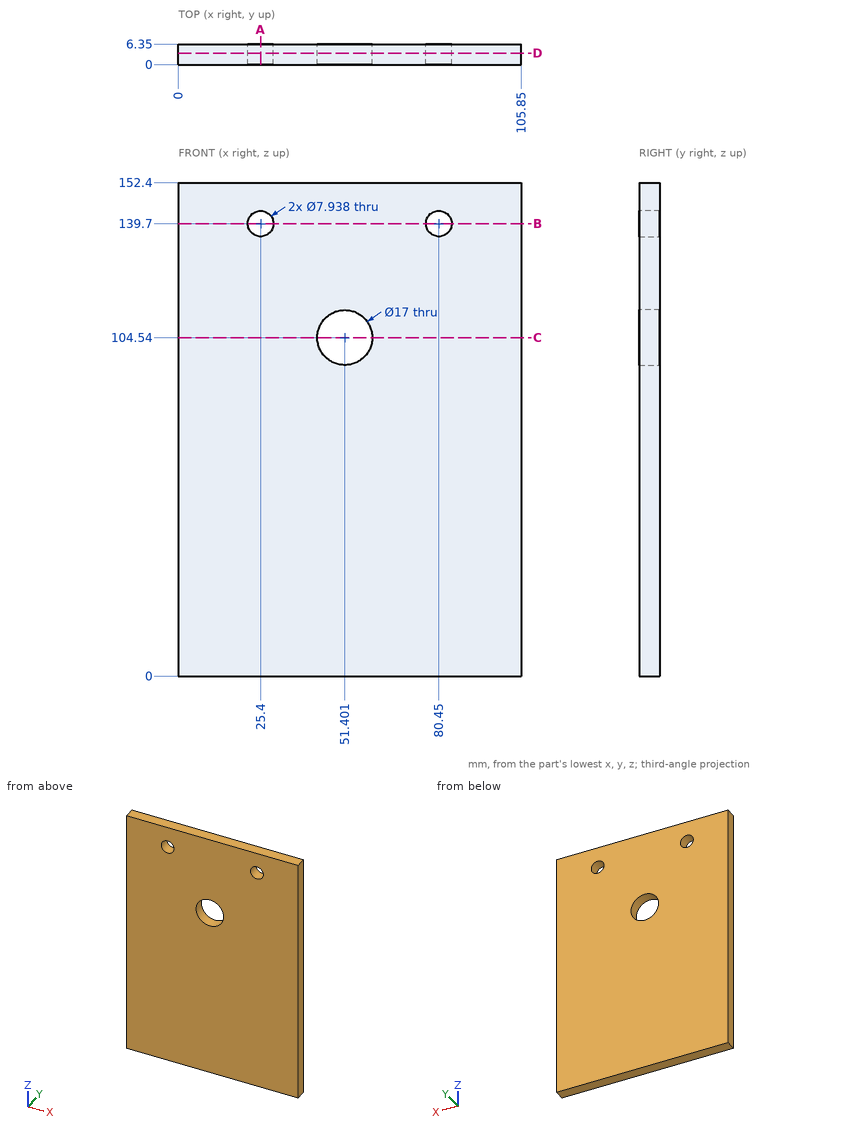
For this review, use the dimensioned drawing (mm, ordinates from the lowest corner) and the shaded views. Give positions to 0.01 mm unless a question says otherwise; leave off trailing zeros. Order: outer loops, then holes, each group sorted by start corner. A loop starts at its lowest first (then second) coordinate and runs counter-clockwise, first axis right, second up.
1) Take a section at B-B (z = 139.7). Give the boundary of the cut face in (x, y).
2) Take a section at C-C (z = 104.54). Give the boundary of the cut face in (x, y), then the cut area to 3 significant figures.
3) Take a section at D-D (y = 3.5). Give the boundary of the cut face in (x, z).
4) Take a section at A-A (x = 25.4). Give the boundary of the cut face in (y, z).
5) Wall thickness on line 1 (X direction, y = 4.25, z = 139.7); line 2 (X direction, y = 2.25, z = 104.54); line 3 (Z direction, x = 80.45, y = 4.5): over which ranges is each line inside the solid? List them lowest first.
6) Insertion check: pin 1 (5 mm diameter, centred on x = 80.45, z = 139.7, fed in from +Y). The pin has a flat end and moves straight along its axis. Give the tip position at first contact, or say it passes through.
Derived:
1. outline: (0, 0) - (21.43, 0) - (21.43, 6.35) - (0, 6.35) - close; (29.37, 0) - (76.48, 0) - (76.48, 6.35) - (29.37, 6.35) - close; (84.42, 0) - (105.85, 0) - (105.85, 6.35) - (84.42, 6.35) - close
2. outline: (0, 0) - (42.9, 0) - (42.9, 6.35) - (0, 6.35) - close; (59.9, 0) - (105.85, 0) - (105.85, 6.35) - (59.9, 6.35) - close
2. area: 564 mm2
3. outline: (0, 0) - (105.85, 0) - (105.85, 152.4) - (0, 152.4) - close; hole circle Ø7.94 at (25.4, 139.7); hole circle Ø17 at (51.4, 104.54); hole circle Ø7.94 at (80.45, 139.7)
4. outline: (0, 0) - (6.35, 0) - (6.35, 135.73) - (0, 135.73) - close; (0, 143.67) - (6.35, 143.67) - (6.35, 152.4) - (0, 152.4) - close
5. line 1: x = 0 to 21.43, 29.37 to 76.48, 84.42 to 105.85
5. line 2: x = 0 to 42.9, 59.9 to 105.85
5. line 3: z = 0 to 135.73, 143.67 to 152.4
6. pin 1: passes through
